The model under review builds one solid part; all positions refer to its coordinate system, in mm. Round coordinates to 2 decimals unless told otherwise and drop trailing zeros. Order: outer loops, then holes, each group sorted by start corner. A loop starts at its lowest first (then second) coordinate and runs counter-clockwise, first axis right, second up. Notation, with made-up numbers: M 81.5,37.5 L 111.5,37.5 A28 ccw 111.5,70.5 Z; hole C 53,56 d1. An arc over 180 degrees is marked long. Answer as a JSON object with one key per item and string values. Group by question number.
1. Mouldability with a two-part tool opening along X and no side actions: class faces 1 (the face through (-32.7, -35.1, 3.1)), 2 (the face through (-41.275, -1, 3)), 3 (the face through (-1, 41.275, 3)) as released by +X, released by -X, zero draft, split by the parting line, or undercut.
2. Add section A-A on x = 0. State the section outline as (y, z) points (3 decimals).
3. Add section C-C on x = -8.5. State the section outline as (y, z) points (3 decimals).
4. To check wall thickness, follow probe 1 along X at (y, z) = (34, 4) (3 decimals); probe 2 along Y at (x, z) = (-16, 2.25) (3 decimals). State the ranges of each line that lie inside material, in increasing order. Write a range as [from, to].
5. Add section B-B on z = 1.75. State the section outline as (x, y) points (3 decimals).
```python
from build123d import *

# Parameters (mm, degrees)
F0_W     = 82.55
F0_H     = 82.55
F0_R     = 1.778
F0_R_2   = 19.05
F1_DEPTH = 6.35


# Not quite as in the source:
# - a length typed as a fraction of an inch, garbled in the dataset ("3 / 203.2 mm" for 3/8 in), is restored


with BuildPart() as f1:
    # F0 (on Top) → F1 (new body)
    with BuildSketch(Plane.XY):
        Rectangle(F0_W, F0_H)
        with Locations((-33.528, -33.528)):
            Circle(F0_R, mode=Mode.SUBTRACT)
        with Locations((33.528, -33.528)):
            Circle(F0_R, mode=Mode.SUBTRACT)
        with Locations((-33.528, 33.528)):
            Circle(F0_R, mode=Mode.SUBTRACT)
        Circle(F0_R_2, mode=Mode.SUBTRACT)
        with Locations((33.528, 33.528)):
            Circle(F0_R, mode=Mode.SUBTRACT)
    extrude(amount=F1_DEPTH)


solid = f1.part
```
Recorded:
{
 "1": {"face 1": "undercut", "face 2": "released by -X", "face 3": "zero draft"},
 "2": {"outline": "M -41.275,0 L -19.05,0 L -19.05,6.35 L -41.275,6.35 Z; M 19.05,0 L 41.275,0 L 41.275,6.35 L 19.05,6.35 Z"},
 "3": {"outline": "M -41.275,0 L -17.049,0 L -17.049,6.35 L -41.275,6.35 Z; M 17.049,0 L 41.275,0 L 41.275,6.35 L 17.049,6.35 Z"},
 "4": {"probe 1": "x = [-41.275, -35.242], [-31.814, 31.814], [35.242, 41.275]", "probe 2": "y = [-41.275, -10.339], [10.339, 41.275]"},
 "5": {"outline": "M -41.275,-41.275 L 41.275,-41.275 L 41.275,41.275 L -41.275,41.275 Z; hole C -33.528,-33.528 d3.556; hole C -33.528,33.528 d3.556; hole C 0,0 d38.1; hole C 33.528,-33.528 d3.556; hole C 33.528,33.528 d3.556"}
}
